Geometry check sheet. Reference: the model listing, model coordinates, mm. A direction names the side the tool comes from. Round coordinates to 2 decimals unless told otherwise and drop trailing zeros. Write each loop counter-clockwise with the first axis right and the second up, starting at its lowest first coordinate (ties: lowest second). Pieces come first, ordered by that corner, then holes. Notation, with made-up numbers: (-23, 64.5) -> (31, 64.5) arc R18 ccw to (31, 83.5) -> close; hole circle Ø11 at (80.25, 43). An arc over 180 degrees is marked (long way). Use a Markdown table: item, result.
Autodesk Inventor part; units mm, degrees
ref_plane "YZ Plane" through (0, 0, 0) normal (1, 0, 0) x (0, 1, 0)
ref_plane "XZ Plane" through (0, 0, 0) normal (0, 1, 0) x (-1, 0, 0)
ref_plane "XY Plane" through (0, 0, 0) normal (0, 0, 1) x (1, 0, 0)
sketch "Sketch1" plane through (0, 0, 0) normal (1, 0, 0) x (0, 1, 0)
  line L0 (0, 0) -> (1.6, 0) construction
  line L1 (1.6, 0) -> (4.95, 0)
  line L2 (4.95, 0) -> (4.95, -1.5)
  line L3 (4.95, -1.5) -> (3.95, -1.5)
  line L4 (3.95, -1.5) -> (3.95, -5)
  line L5 (3.95, -5) -> (1.6, -5)
  line L6 (1.6, -5) -> (1.6, 0)
  line L7 (0, 0) -> (0, -13.7466) construction
  dimension "d0" = 1.6
  dimension "d1" = 3.95
  dimension "d2" = 1
  dimension "d3" = 1.5
  dimension "d4" = 3.5
revolve "Revolution1" add sketch "Sketch1" angle 360 about axis through (0, 0, 0) along (0, 0, -1)
sketch "Sketch2" plane through (0, 0, 0) normal (0, 0, 1) x (1, 0, 0)
  line L0 (2.85, -2.85) -> (-2.85, -2.85)
  line L1 (-2.85, -2.85) -> (-2.85, 2.85)
  line L2 (-2.85, 2.85) -> (2.85, 2.85)
  line L3 (2.85, 2.85) -> (2.85, -2.85)
  line L4 (2.85, -2.85) -> (-2.85, 2.85) construction
  line L5 (-2.85, -2.85) -> (2.85, 2.85) construction
  point P0 (0, 0)
  dimension "d6" = 5.7
extrude "Extrusion1" cut sketch "Sketch2" against normal blind 2.7
fillet "Fillet1" radius 0.5 2 edges at (0, -3.95, -5) (0, -1.6, -5)
properties part number "HD_BearingShaft1"
(1) Section check A-A on x = 0. Record the cut outline in (y, z), plus the area to 3 significant figures.
A:
| item | result |
|---|---|
| outline | (-4.95, -1.5) -> (-3.95, -1.5) -> (-3.95, -4.5) arc R0.5 ccw to (-3.45, -5) -> (-2.1, -5) arc R0.5 ccw to (-1.6, -4.5) -> (-1.6, -2.7) -> (-2.85, -2.7) -> (-2.85, 0) -> (-4.95, 0) -> close; (1.6, -4.5) arc R0.5 ccw to (2.1, -5) -> (3.45, -5) arc R0.5 ccw to (3.95, -4.5) -> (3.95, -1.5) -> (4.95, -1.5) -> (4.95, 0) -> (2.85, 0) -> (2.85, -2.7) -> (1.6, -2.7) -> close |
| area | 19.5 mm2 |
(2) Thickness scan on line 1 (Y direction, x = 0, z = -3.95); line 2 (Y direction, x = -1, z = -1.3). Record the ranges inside material, lowest first.
A:
| item | result |
|---|---|
| line 1 | y = -3.95 to -1.6, 1.6 to 3.95 |
| line 2 | y = -4.85 to -2.85, 2.85 to 4.85 |
(3) Section check C-C on z = -0.65. Record the cut outline in (x, y), plus the area to 3 significant figures.
A:
| item | result |
|---|---|
| outline | circle Ø9.9 at (0, 0); hole (-2.85, -2.85) -> (2.85, -2.85) -> (2.85, 2.85) -> (-2.85, 2.85) -> close |
| area | 44.5 mm2 |
(4) Section check D-D on z = -2.55. Record the cut outline in (x, y).
A:
| item | result |
|---|---|
| outline | (-2.85, -2.73) -> (-2.85, 2.73) arc R3.95 ccw to start; (-2.73, -2.85) arc R3.95 ccw to (2.73, -2.85) -> close; (-2.73, 2.85) -> (2.73, 2.85) arc R3.95 ccw to start; (2.85, -2.73) arc R3.95 ccw to (2.85, 2.73) -> close |
(5) Release check for a two-part mould opening along X. For faces 4 (the face through (-1, -4, -1.5)), 5 (the face through (1.49, 4.72, -0.76)), 6 (the face through (0.97, -1.27, -3.59)), 7 (the face through (0, -2.85, -1)) record: +X half, -X half, draft (parallel to the pull), parting line (faces both ways), or undercut.
A:
| item | result |
|---|---|
| face 4 | draft |
| face 5 | parting line |
| face 6 | undercut |
| face 7 | undercut |
(6) Gauge pin test, flat ends, axial feed: pin 1 Ø3 at (x, z) = (-1.5, -2) entering from -Y; pin 2 Ø4.5 at (x, y) = (0, -0.5) entering from +Z; pin 3 Ø3.5 at (x, y) = (0, 0) entering from -Z; pin 4 Ø1 at (x, z) = (1, -3) entering from -Y. Record the tip position at first contact, or that the pin passes through.
A:
| item | result |
|---|---|
| pin 1 | stops at y = -4.95 |
| pin 2 | stops at z = -2.7 |
| pin 3 | stops at z = -4.86 |
| pin 4 | stops at y = -3.92 |
(7) Access from +Z, -Z, +X, -X, +Y, -Y to the whole of each face (thin tool, end or side, straight path). Record for faces 1 (the face through (0, 2.85, -1)), 2 (the face through (-2.3, 0, -5)), 3 (the face through (-2.404, -3.135, -3.021)).
A:
| item | result |
|---|---|
| face 1 | +Z |
| face 2 | -Z, +X, -X, +Y, -Y |
| face 3 | -Z |
